Check sheet for the modelled part. Datum: model origin and axes. Units: mm. Face numbers are marked on the shaded views. A direction names the side the tool comes from. Give positions to 0.01 mm unless a question says otherwise; leave off trailing zeros. Order: outer loops, then holes, each group sorted by start corner. A loop starts at its lowest first (then second) coordinate and runs counter-clockwise, first axis right, second up.
Item 1: Material ranges on line 1 along X through (y, z) = (14.75, 0); line 2 along Z through (x, y) = (0, 0.7); line 3 along X through (y, z) = (0.8, 4.44), recorded low to high.
Item 2: Release check for a two-part mould opening along X. For the marked faces 1, 2 and 3 record: released by +X, released by -X, zero draft, split by the parting line, or undercut.
Item 3: Access from +Z, -Z, +X, -X, +Y, -Y to the whole of each face (thin tool, end or side, straight path). Record for the marked faces 4, 5 and 6.
Item 4: Gauge pin test, flat ends, axial feed: P1, Ø2, axis at x = -1.5, z = 9, coming from the +Y side; P2, Ø3, axis at x = 0, z = -8.88, coming from the +Y side; P3, Ø3, axis at x = 2, z = 1.5, coming from the +Y side; P4, Ø8, axis at x = -5, y = 2, coming from the -Z side. Record the tip position at first contact, or that the pin passes through.
Item 5: Sectioned sample at C-C on z = 0. Record the boundary of the cut face in (x, y) (3 decimals).
Item 6: Sectioned sample at B-B on z = -8.88. Record the boundary of the cut face in (x, y), and give its area (3 significant figures).
Item 7: Sectioned sample at A-A on x = 0. Record the boundary of the cut face in (y, z) (3 decimals), and give its area (3 significant figures).
Item 8: Sectioned sample at D-D on x = 8.75. Record the boundary of the cut face in (y, z), and give its area (3 significant figures).
from build123d import *

# Parameters (mm, degrees)
SKETCH1_R           = 6.22
BOSS_EXTRUDE1_DEPTH = 15
SKETCH2_R           = 11.93
BOSS_EXTRUDE2_DEPTH = 1.2
CUT_EXTRUDE1_REACH  = 3.2
SKETCH3_R           = 1.6
SKETCH4_R           = 4.92
CUT_EXTRUDE2_DEPTH  = 0.93
SKETCH5_R           = 4.875
BOSS_EXTRUDE3_DEPTH = 0.76
SKETCH6_R           = 2.425
BOSS_EXTRUDE4_DEPTH = 1.88
SKETCH7_R           = 5.445
SKETCH7_R_2         = 4.875
CUT_EXTRUDE3_DEPTH  = 0.25


with BuildPart() as part:
    # Sketch1 → Boss-Extrude1 (new body)
    with BuildSketch(Plane(origin=(0, 0, 0), x_dir=(1, 0, 0), z_dir=(0, 1, 0))):
        Circle(SKETCH1_R)
    extrude(amount=BOSS_EXTRUDE1_DEPTH)

    # Sketch2 → Boss-Extrude2 (add)
    with BuildSketch(Plane.XZ):
        Circle(SKETCH2_R)
    extrude(amount=-BOSS_EXTRUDE2_DEPTH)

    # Sketch3 → Cut-Extrude1 (cut, up to next)
    with BuildSketch(Plane(origin=(0, 1.2, 0), x_dir=(1, 0, 0), z_dir=(0, 1, 0)), mode=Mode.PRIVATE) as cut_extrude1_sk1:
        with Locations((0, 8.88)):
            Circle(SKETCH3_R)
    cut_extrude1_tool1 = extrude(cut_extrude1_sk1.sketch, amount=-CUT_EXTRUDE1_REACH, mode=Mode.PRIVATE) & part.part
    add(cut_extrude1_tool1.solids().sort_by_distance((0, 1.2, -8.88))[0], mode=Mode.SUBTRACT)
    # Sketch3 → Cut-Extrude1 (cut, up to next)
    with BuildSketch(Plane(origin=(0, 1.2, 0), x_dir=(1, 0, 0), z_dir=(0, 1, 0)), mode=Mode.PRIVATE) as cut_extrude1_sk2:
        with Locations((7.690305586, -4.44)):
            Circle(SKETCH3_R)
    cut_extrude1_tool2 = extrude(cut_extrude1_sk2.sketch, amount=-CUT_EXTRUDE1_REACH, mode=Mode.PRIVATE) & part.part
    add(cut_extrude1_tool2.solids().sort_by_distance((7.690306, 1.2, 4.44))[0], mode=Mode.SUBTRACT)
    # Sketch3 → Cut-Extrude1 (cut, up to next)
    with BuildSketch(Plane(origin=(0, 1.2, 0), x_dir=(1, 0, 0), z_dir=(0, 1, 0)), mode=Mode.PRIVATE) as cut_extrude1_sk3:
        with Locations((-7.690305586, -4.44)):
            Circle(SKETCH3_R)
    cut_extrude1_tool3 = extrude(cut_extrude1_sk3.sketch, amount=-CUT_EXTRUDE1_REACH, mode=Mode.PRIVATE) & part.part
    add(cut_extrude1_tool3.solids().sort_by_distance((-7.690306, 1.2, 4.44))[0], mode=Mode.SUBTRACT)

    # Sketch4 → Cut-Extrude2 (cut)
    with BuildSketch(Plane(origin=(0, 15, 0), x_dir=(1, 0, 0), z_dir=(0, 1, 0))):
        Circle(SKETCH4_R)
    extrude(amount=-CUT_EXTRUDE2_DEPTH, mode=Mode.SUBTRACT)

    # Sketch5 → Boss-Extrude3 (add)
    with BuildSketch(Plane.XZ):
        Circle(SKETCH5_R)
    extrude(amount=BOSS_EXTRUDE3_DEPTH)

    # Sketch6 → Boss-Extrude4 (add)
    with BuildSketch(Plane.XZ.offset(0.76)):
        Circle(SKETCH6_R)
    extrude(amount=BOSS_EXTRUDE4_DEPTH)

    # Sketch7 → Cut-Extrude3 (cut)
    with BuildSketch(Plane.XZ):
        Circle(SKETCH7_R)
        Circle(SKETCH7_R_2, mode=Mode.SUBTRACT)
    extrude(amount=-CUT_EXTRUDE3_DEPTH, mode=Mode.SUBTRACT)


solid = part.part
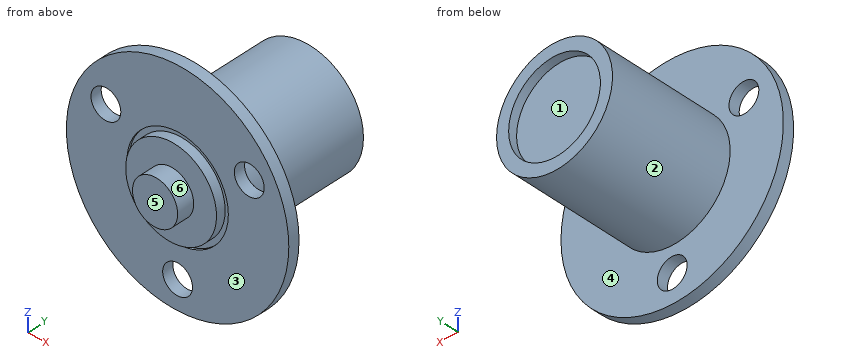
Report:
1. line 1: x = -6.22 to -4.92, 4.92 to 6.22
1. line 2: z = -11.93 to -10.48, -7.28 to 11.93
1. line 3: x = -11.07 to -9.29, -6.09 to 6.09, 9.29 to 11.07
2. face 1: undercut
2. face 2: split by the parting line
2. face 3: zero draft
3. face 4: +Y
3. face 5: +Z, -Z, +X, -X, -Y
3. face 6: -Y
4. P1: stops at y = 1.2
4. P2: passes through
4. P3: stops at y = 14.07
4. P4: stops at z = -11.88
5. outline: (-11.93, 0) - (-5.445, 0) - (-5.445, 0.25) - (-4.875, 0.25) - (-4.875, -0.76) - (-2.425, -0.76) - (-2.425, -2.64) - (2.425, -2.64) - (2.425, -0.76) - (4.875, -0.76) - (4.875, 0.25) - (5.445, 0.25) - (5.445, 0) - (11.93, 0) - (11.93, 1.2) - (6.22, 1.2) - (6.22, 15) - (4.92, 15) - (4.92, 14.07) - (-4.92, 14.07) - (-4.92, 15) - (-6.22, 15) - (-6.22, 1.2) - (-11.93, 1.2) - close
6. outline: (-7.97, 0) - (-1.6, 0) - (-1.6, 1.2) - (-7.97, 1.2) - close; (1.6, 0) - (7.97, 0) - (7.97, 1.2) - (1.6, 1.2) - close
6. area: 15.3 mm2
7. outline: (-2.64, -2.425) - (-0.76, -2.425) - (-0.76, -4.875) - (0.25, -4.875) - (0.25, -5.445) - (0, -5.445) - (0, -7.28) - (1.2, -7.28) - (1.2, -6.22) - (15, -6.22) - (15, -4.92) - (14.07, -4.92) - (14.07, 4.92) - (15, 4.92) - (15, 6.22) - (1.2, 6.22) - (1.2, 11.93) - (0, 11.93) - (0, 5.445) - (0.25, 5.445) - (0.25, 4.875) - (-0.76, 4.875) - (-0.76, 2.425) - (-2.64, 2.425) - close; (0, -11.93) - (1.2, -11.93) - (1.2, -10.48) - (0, -10.48) - close
7. area: 204 mm2
8. outline: (0, -8.11) - (1.2, -8.11) - (1.2, 3.24) - (0, 3.24) - close; (0, 5.64) - (1.2, 5.64) - (1.2, 8.11) - (0, 8.11) - close
8. area: 16.6 mm2
